Read the model definition and answer for the solid it produces. Units are mm, in the model's axes. Give positions to 0.01 mm unless a question says otherwise; leave off trailing zeros. Loops run counter-clockwise (first coordinate to the right, second up) from the corner with the lowest first, then second, coordinate; pieces in that order, holes last. Notation, with made-up numbers: (80.25, 19) - (89.25, 19) arc R22 ccw to (89.25, 44) - close; hole circle Ø9 at (79.25, -36.75). An arc over 180 degrees is marked (long way). Put each result on its own line as item: value. Start each with the question number.
1. A cutting plane is placed at B-B, the plane y = 18. Determine the outline of the cut face in (x, z), plus the area to 3 significant figures.
2. A cutting plane is placed at C-C, the plane z = 8.5. Count the separate pieces of the cut face and the enclosed holes in it, plus the area to 3 significant figures.
3. Consider L1, parallel to X at y = 43, z = 1.75; L2, parallel to X at y = 17, z = 1.25; L3, parallel to Y at x = 66.5, z = 8.5. Determine where each line is inside the solid, lowest interval first. Write a range as from..to.
4. Given pin 1 Ø4 at (y, z) = (53, 3.5) entering from +X; pin 2 Ø3 at (x, z) = (7.5, 4) entering from +Y; pin 3 Ø5 at (y, z) = (29.5, 7) entering from -X, each flat-ended and moving along its own axis, determine where each tip first touches the part or whether it passes through.
5. A cutting plane is placed at A-A, the plane x = 127.5. Determine the outline of the cut face in (y, z), plus the area to 3 significant figures.
6. A cutting plane is placed at D-D, the plane y = 34.5. Determine the outline of the cut face in (x, z).
Autodesk Inventor part; units mm, degrees
ref_plane "YZ Plane" through (0, 0, 0) normal (1, 0, 0) x (0, 1, 0)
ref_plane "XZ Plane" through (0, 0, 0) normal (0, 1, 0) x (-1, 0, 0)
ref_plane "XY Plane" through (0, 0, 0) normal (0, 0, 1) x (1, 0, 0)
sketch "Sketch1" plane through (0, 0, 0) normal (0, 0, 1) x (1, 0, 0)
  line L0 (0, 0) -> (180, 0)
  line L1 (180, 0) -> (180, 80)
  line L2 (180, 80) -> (0, 80)
  line L3 (0, 80) -> (0, 0)
  dimension "d0" = 180
  dimension "d1" = 80
extrude "Extrusion1" add sketch "Sketch1" along normal blind 10.4
sketch "Sketch2" plane through (0, 0, 10.4) normal (0, 0, 1) x (1, 0, 0)
  line L0 (0, 80) -> (0, 0)
  line L1 (0, 60) -> (10, 60)
  line L2 (10, 60) -> (10, 20)
  line L3 (10, 20) -> (0, 20)
  line L4 (0, 9.6) -> (10, 9.6)
  line L5 (10, 9.6) -> (10, 0)
  line L6 (0, 0) -> (180, 0)
  line L7 (0, 70.4) -> (10, 70.4)
  line L8 (10, 70.4) -> (10, 80)
  line L9 (180, 80) -> (0, 80)
  line L10 (170, 80) -> (170, 70.4)
  line L11 (170, 70.4) -> (180, 70.4)
  line L12 (180, 0) -> (180, 80)
  line L13 (180, 60) -> (170, 60)
  line L14 (170, 60) -> (170, 20)
  line L15 (170, 20) -> (180, 20)
  line L16 (170, 0) -> (170, 9.6)
  line L17 (170, 9.6) -> (180, 9.6)
  line L18 (162, 64) -> (162, 16)
  line L19 (18, 16) -> (18, 64)
  line L20 (112, 64) -> (112, 16)
  line L21 (68, 16) -> (68, 64)
  line L22 (18, 64) -> (68, 64)
  line L23 (112, 64) -> (162, 64)
  line L24 (162, 16) -> (112, 16)
  line L25 (68, 16) -> (18, 16)
  line L26 (93.25, 12) -> (93.25, 68)
  line L27 (86.75, 12) -> (86.75, 68)
  arc A0 (86.75, 12) -> (93.25, 12) centre (90, 12) ccw
  arc A1 (93.25, 68) -> (86.75, 68) centre (90, 68) ccw
  dimension "d4" = 40
  dimension "d5" = 10.4
  dimension "d6" = 10.4
  dimension "d7" = 9.6
  dimension "d8" = 10
  dimension "d9" = 40
  dimension "d10" = 10.4
  dimension "d11" = 10.4
  dimension "d13" = 10
  dimension "d14" = 10
  dimension "d15" = 9.6
  dimension "d19" = 8
  dimension "d21" = 8
  dimension "d22" = 50
  dimension "d23" = 50
  dimension "d24" = 16
  dimension "d25" = 16
  dimension "d26" = 16
  dimension "d27" = 16
  dimension "d31" = 12
  dimension "d32" = 12
  dimension "d33" = 6.5
  dimension "d34" = 18.75
extrude "Extrusion2" cut sketch "Sketch2" against normal up to next contours L9 L8 L7 L0 | L1 L2 L3 L0 | L9 L12 L11 L10 | L4 L5 L6 L0 | L12 L15 L14 L13 | L16 L17 L12 L6 | L18 L24 L20 L23 | L19 L22 L21 L25 | A0 L27 A1 L26
equation "\"d24\" = d26"
equation "\"d25\" = d26"
equation "\"d27\" = d26"
properties part number "center mount"
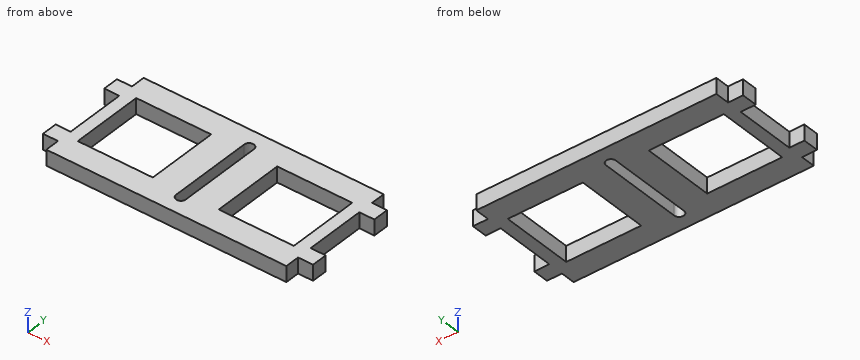
Return value:
1. outline: (0, 0) - (18, 0) - (18, 10.4) - (0, 10.4) - close; (68, 0) - (86.75, 0) - (86.75, 10.4) - (68, 10.4) - close; (93.25, 0) - (112, 0) - (112, 10.4) - (93.25, 10.4) - close; (162, 0) - (180, 0) - (180, 10.4) - (162, 10.4) - close
1. area: 764 mm2
2. separate pieces: 1
2. enclosed holes: 3
2. area: 8,020 mm2
3. L1: x = 10..18, 68..86.75, 93.25..112, 162..170
3. L2: x = 0..18, 68..86.75, 93.25..112, 162..180
3. L3: y = 0..16, 64..80
4. pin 1: stops at x = 170
4. pin 2: stops at y = 70.4
4. pin 3: stops at x = 10
5. outline: (0, 0) - (16, 0) - (16, 10.4) - (0, 10.4) - close; (64, 0) - (80, 0) - (80, 10.4) - (64, 10.4) - close
5. area: 333 mm2
6. outline: (10, 0) - (18, 0) - (18, 10.4) - (10, 10.4) - close; (68, 0) - (86.75, 0) - (86.75, 10.4) - (68, 10.4) - close; (93.25, 0) - (112, 0) - (112, 10.4) - (93.25, 10.4) - close; (162, 0) - (170, 0) - (170, 10.4) - (162, 10.4) - close
